Source: three-view drawing plus pictorial views. Frame: mm from the lowest corner of the part. A direction names the side the tool comes from. Give positions to 0.01 mm unless a question says otherwise; leave off trailing zeros. Write each loop counter-clockwise with the first axis right and the second up, starting at its lowest first coordinate (ties: lowest second). Pieces come first, ordered by that corner, then holes.
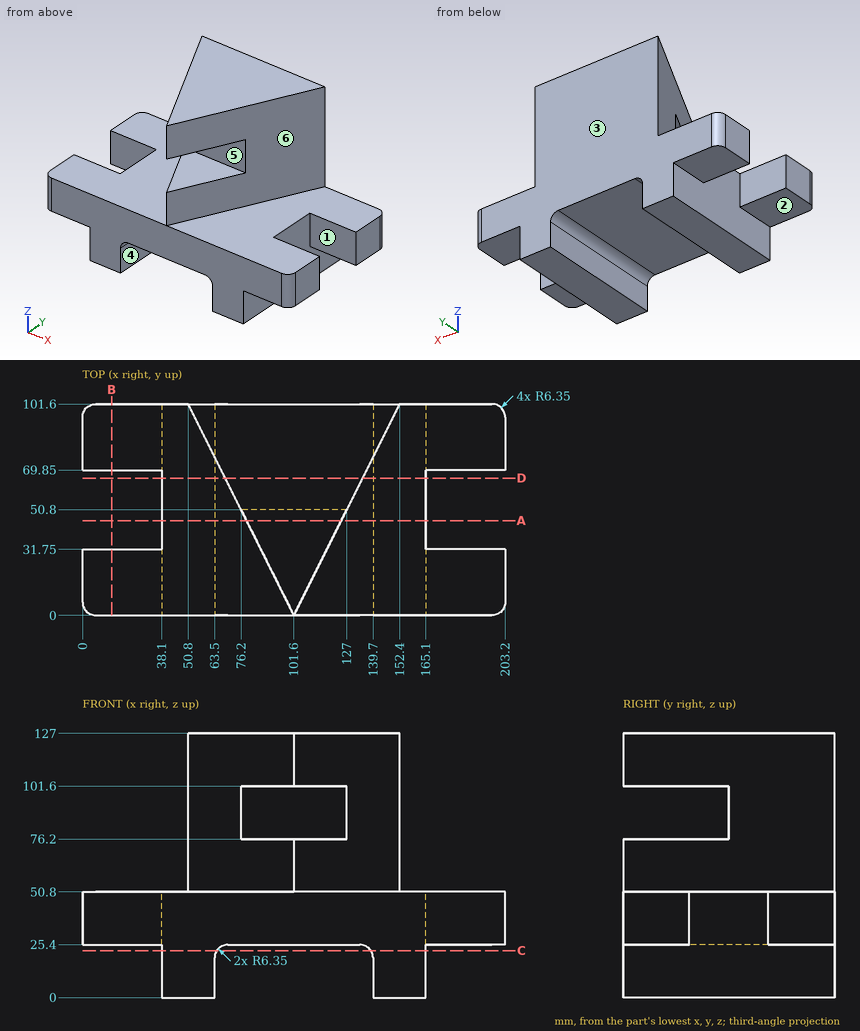
Q1. Pull-direction query (Y, two-part tool) for the marked faces 1, 2 and 3; classes: released by +Y, released by -Y, zero draft, split by the parting line, or undercut.
Filled sheet:
face 1: undercut
face 2: zero draft
face 3: released by +Y
Q2. Section B-B on x = 14. Output: boundary loops of the cut face in (y, z).
Filled sheet:
outline: (0, 25.4) - (31.75, 25.4) - (31.75, 50.8) - (0, 50.8) - close; (69.85, 25.4) - (101.6, 25.4) - (101.6, 50.8) - (69.85, 50.8) - close
Q3. Section D-D on y = 66. Output: boundary loops of the cut face in (x, z), plus the area to 3 significant figures.
Filled sheet:
outline: (38.1, 0) - (63.5, 0) - (63.5, 19.05) arc R6.35 cw to (69.85, 25.4) - (133.35, 25.4) arc R6.35 cw to (139.7, 19.05) - (139.7, 0) - (165.1, 0) - (165.1, 50.8) - (134.6, 50.8) - (134.6, 127) - (68.6, 127) - (68.6, 50.8) - (38.1, 50.8) - close
area: 9,560 mm2
Q4. Ray query, line 1 along Z through (x, y) = (99, 35.5); line 2 along Z through (x, y) = (159.5, 90); line 3 along Y through (x, z) = (27, 43.5). Return the intervals inside material, ascending.
Filled sheet:
line 1: z = 25.4 to 76.2, 101.6 to 127
line 2: z = 0 to 50.8
line 3: y = 0 to 31.75, 69.85 to 101.6
Q5. Pin query (flat end, axial travel): P1, Ø4, axis at x = 53, y = 81.5, coming from the -Z side; P2, Ø19, axis at x = 94, y = 29.5, coming from the -Z side; P3, Ø15, axis at y = 40, z = 26.5, coming from the -X side; P4, Ø21, axis at y = 61.5, z = 8, coming from the +X side. Return the tip coordinate at first contact, or that it passes through.
Filled sheet:
P1: stops at z = 0
P2: stops at z = 25.4
P3: stops at x = 38.1
P4: stops at x = 165.1
Q6. Access query for the marked faces 4, 5 and 6. Directions: +Z, -Z, +X, -X, +Y, -Y. A direction counts if a zero-diameter tool reaches every point of the face in a straight line with its end or side. Return the directions, or none.
Filled sheet:
face 4: -Z, +Y, -Y
face 5: +X, -X, -Y
face 6: +Z, +X, -Y
Q7. Section C-C on z = 22.5. Output: boundary loops of the cut face in (x, y).
Filled sheet:
outline: (38.1, 0) - (64.52, 0) - (64.52, 101.6) - (38.1, 101.6) - close; (138.68, 0) - (165.1, 0) - (165.1, 101.6) - (138.68, 101.6) - close
Q8. Section A-A on y = 45.5. Output: boundary loops of the cut face in (x, z).
Filled sheet:
outline: (38.1, 0) - (63.5, 0) - (63.5, 19.05) arc R6.35 cw to (69.85, 25.4) - (133.35, 25.4) arc R6.35 cw to (139.7, 19.05) - (139.7, 0) - (165.1, 0) - (165.1, 50.8) - (124.35, 50.8) - (124.35, 76.2) - (78.85, 76.2) - (78.85, 50.8) - (38.1, 50.8) - close; (78.85, 101.6) - (124.35, 101.6) - (124.35, 127) - (78.85, 127) - close
